Drawing for the job (mm, zero at the part's lowest x, y, z). A direction names the side the tool comes from. Give positions to 0.01 mm unless a question says otherwise; leave off trailing zeros. Loops run counter-clockwise (first coordinate to the right, second up) from the corner with the lowest first, then second, coordinate; pieces in that order, holes last. Notation, with made-up numbers: (-37, -10.75) -> (21, -10.75) arc R19 cw to (21, 12.25) -> close; hole circle Ø10 at (52, 18). An arc over 180 degrees is marked (long way). Use CSV: the item, a comma, the result in double quotes. Start each with the question number.
(1) Cut at C-C on z = 1.3. Write the cut outline in (x, y), then the cut area to 3 significant figures.
(2) Cut at A-A on y = 9.3. Write the cut outline in (x, z).
(3) Cut at D-D on x = 1.5. Write the cut outline in (y, z), then the cut area to 3 significant figures.
(4) 3-axis set-ups, long thin cutter, end or side, ignore diameter. For the marked faces 1, 2 and 3: which of +Z, -Z, +X, -X, +Y, -Y reach the whole face in a straight line?
(5) Drill centre lines: probe 1 along Y at (x, z) = (9.3, 2.85); probe 2 along Y at (x, z) = (9.3, 1.75); probe 3 along Z at (x, y) = (6, 6.75). Where is each one in solid material? Low to high.
(6) Flat gauge pins, fed straight in: pin 1 (2 mm diameter, centred on x = 6, y = 7.5, fed in from -Z); pin 2 (10 mm diameter, centred on x = 14, y = 12, fed in from -Z); pin 3 (1.5 mm diameter, centred on y = 12.5, z = 1.5, fed in from +X). Where does each tip first touch, or does it go through?
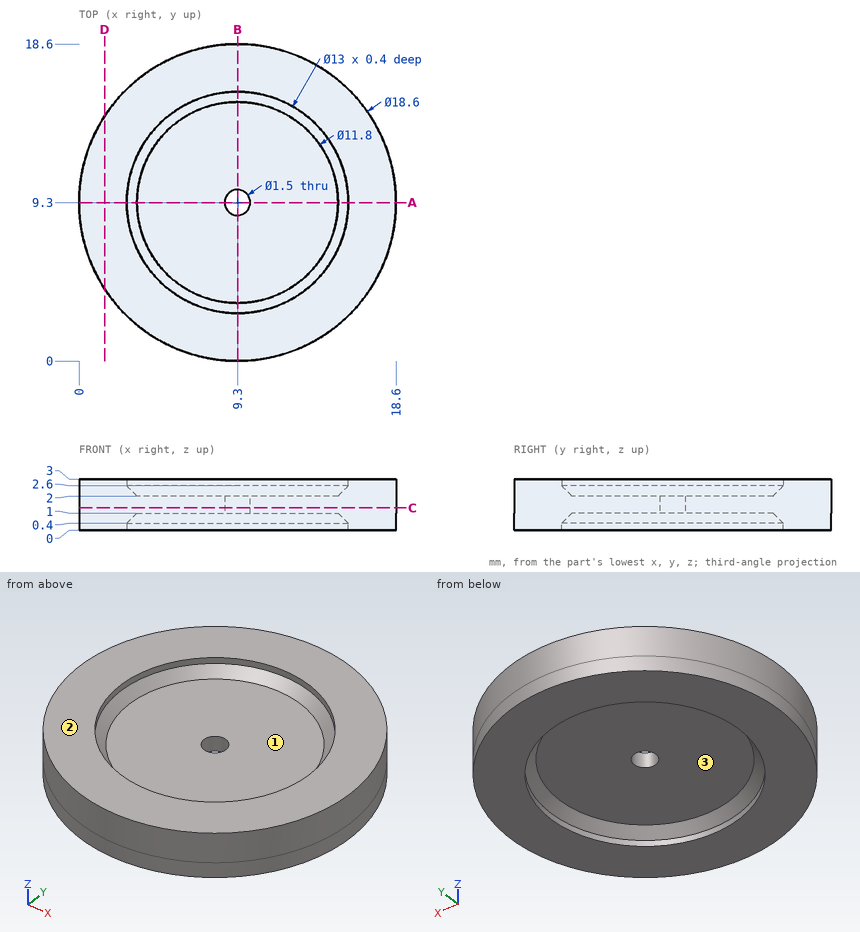
Check result:
1,outline,"circle Ø18.6 at (9.3, 9.3); hole circle Ø1.5 at (9.3, 9.3)"
1,area,"270 mm²"
2,outline,"(0, 0) -> (2.8, 0) -> (2.8, 0.4) -> (3.4, 1) -> (8.55, 1) -> (8.55, 2) -> (3.4, 2) -> (2.8, 2.6) -> (2.8, 3) -> (0, 3) -> close; (10.05, 1) -> (15.2, 1) -> (15.8, 0.4) -> (15.8, 0) -> (18.6, 0) -> (18.6, 3) -> (15.8, 3) -> (15.8, 2.6) -> (15.2, 2) -> (10.05, 2) -> close"
3,outline,"(4.24, 0) -> (14.36, 0) -> (14.36, 3) -> (4.24, 3) -> close"
3,area,"30.4 mm²"
4,face 1,"+Z"
4,face 2,"+Z, +X, -X, +Y, -Y"
4,face 3,"-Z"
5,probe 1,"0 to 2.8, 15.8 to 18.6"
5,probe 2,"0 to 8.55, 10.05 to 18.6"
5,probe 3,"1 to 2"
6,pin 1,"z = 1"
6,pin 2,"z = 0"
6,pin 3,"x = 18.27"
